from build123d import *
from build123d.topology import SkipClean

# Parameters (mm, degrees)
SKETCH1_R                 = 13.75
SKETCH1_R_2               = 6
BOSS_EXTRUDE1_DEPTH       = 12
SKETCH2_R                 = 13.75
SKETCH2_R_2               = 4.01
BOSS_EXTRUDE3_DEPTH       = 10.98
SKETCH3_R                 = 30
BOSS_EXTRUDE4_DEPTH       = 11.02
F_4_0MM_DOWEL_HOLE1_D     = 4
F_4_0MM_DOWEL_HOLE1_DEPTH = 25.4
F_4_0MM_DOWEL_HOLE1_TIP   = 1.201721238
SKETCH11_W                = 4.05
SKETCH11_H                = 4.3
CUT_EXTRUDE1_DEPTH        = 10
CUT_EXTRUDE2_START        = -32
SKETCH15_R                = 4.01
CUT_EXTRUDE2_DEPTH        = 32
SKETCH16_R                = 13.810706785
SKETCH16_R_2              = 3.943549935
BOSS_EXTRUDE5_DEPTH       = 11


with BuildPart() as part:
    # Sketch1 → Boss-Extrude1 (new body)
    with BuildSketch(Plane(origin=(0, 0, 0), x_dir=(0, 0, -1), z_dir=(1, 0, 0))):
        Circle(SKETCH1_R)
        Circle(SKETCH1_R_2, mode=Mode.SUBTRACT)
    extrude(amount=BOSS_EXTRUDE1_DEPTH)

    # Sketch2 → Boss-Extrude3 (add)
    with BuildSketch(Plane(origin=(12, 0, 0), x_dir=(0, 0, -1), z_dir=(1, 0, 0))):
        with Locations(Location((0, 0, 0), (0, 0, 180))):
            Circle(SKETCH2_R)
        with Locations(Location((0, 0, 0), (0, 0, 180))):
            Circle(SKETCH2_R_2, mode=Mode.SUBTRACT)
    extrude(amount=BOSS_EXTRUDE3_DEPTH)

    # Sketch3 → Boss-Extrude4 (add)
    with BuildSketch(Plane(origin=(22.98, 0, 0), x_dir=(0, 0, -1), z_dir=(1, 0, 0))):
        with Locations(Location((0, 0, 0), (0, 0, 180))):
            Circle(SKETCH3_R)
    extrude(amount=BOSS_EXTRUDE4_DEPTH)

    # Ø4.0mm Dowel Hole1
    with Locations(Plane(origin=(34, 0, 0), x_dir=(0, 0, -1), z_dir=(1, 0, 0))):
        with Locations((-21.643670313, 10.843162234), (-2.353154811, 24.568381237), (19.178491269, 14.724914261), (21.419621846, -8.843771717), (-19.402539736, -12.725523744), (2.129106344, -22.56899072)):
            Hole(F_4_0MM_DOWEL_HOLE1_D / 2, depth=F_4_0MM_DOWEL_HOLE1_DEPTH)
            with Locations((0, 0, -(F_4_0MM_DOWEL_HOLE1_DEPTH + F_4_0MM_DOWEL_HOLE1_TIP / 2))):  # 118° drill point
                Cone(0, F_4_0MM_DOWEL_HOLE1_D / 2, F_4_0MM_DOWEL_HOLE1_TIP, mode=Mode.SUBTRACT)

    # Sketch11 → Cut-Extrude1 (cut)
    with BuildSketch(Plane.ZY):
        with Locations((0, 6)):
            Rectangle(SKETCH11_W, SKETCH11_H)
    extrude(amount=-CUT_EXTRUDE1_DEPTH, mode=Mode.SUBTRACT)

    # Sketch14 → Ø4.0mm Dowel Hole2 (revolve, cut)
    with BuildSketch(Plane(origin=(5, 8.15, 0), x_dir=(0, 0, -1), z_dir=(1, 0, 0))):
        Polygon((0, 0), (0, 26.601721238), (2, 25.4), (2, 0), align=None)
    revolve(axis=Axis((5, 1.8, 0), (0, 1, 0)), mode=Mode.SUBTRACT)

    # Sketch15 → Cut-Extrude2 (cut)
    with SkipClean():  # the faces are left unmerged after this step: merging them gives an invalid solid
        with BuildSketch(Plane(origin=(34, 0, 0), x_dir=(0, 0, -1), z_dir=(1, 0, 0)).offset(CUT_EXTRUDE2_START)):
            Circle(SKETCH15_R)
        extrude(amount=CUT_EXTRUDE2_DEPTH, mode=Mode.SUBTRACT)
    add(part.part.scale(1), mode=Mode.REPLACE)  # the faces are merged on a copy

    # Sketch16 → Boss-Extrude5 (add)
    with BuildSketch(Plane(origin=(34, 0, 0), x_dir=(0, 0, -1), z_dir=(1, 0, 0))):
        with Locations(Location((0, 0, 0), (0, 0, 180))):
            Circle(SKETCH16_R)
        with Locations(Location((0, 0.056450065, 0), (0, 0, 180))):
            Circle(SKETCH16_R_2, mode=Mode.SUBTRACT)
    extrude(amount=BOSS_EXTRUDE5_DEPTH)


solid = part.part
Geometry check sheet. Reference: the model listing, model coordinates, mm. A direction names the side the tool comes from. Round coordinates to 2 decimals unless told otherwise and drop trailing zeros. Loops run counter-clockwise (first coordinate to the right, second up) from the corner with the lowest first, then second, coordinate; pieces in that order, holes last. Notation, with made-up numbers: (20, 13.5) -> (45, 13.5) arc R20 ccw to (45, 30.5) -> close; hole circle Ø3 at (58, 45). An arc over 180 degrees is marked (long way). Answer as a JSON object with one key per item and string values. Group by question number.
Item 1: Cross-section at D-D, the plane y = 18. Record the cut outline in (x, z), plus the area to 3 significant figures.
Item 2: Thickness scan on line 1 along Y through (x, z) = (28.5, -20); line 2 along X through (y, z) = (10.75, 0); line 3 along Y through (x, z) = (25, -2). Record the ranges inside material, lowest first.
Item 3: Release check for a two-part mould opening along Y. For faces 5 (the face through (28.4, -7.5, -22.9)), 6 (the face through (3.8, 8.15, -1.8)), 7 (the face through (22.98, 0, -14)), 8 (the face through (39.423, -4.148, 13.173)) record: pulls with the +Y half, pulls with the -Y half, needs draft (parallel to the pull), parting line crosses it, or undercut.
Item 4: Cross-section at B-B, the plane x = 5. Record the cut outline in (y, z) (3 decimals), plus the area to 3 significant figures.
Item 5: Cross-section at A-A, the plane z = -22. Record the cut outline in (x, y).
Item 6: Cross-section at C-C, the plane x = 19. Record the cut outline in (y, z).
Item 7: Set-up check for faces 1 (the face through (7, 11, 0)), 2 (the face through (45, 3, 3)), 3 (the face through (34, 13, 6)), 4 (the face through (10, 7, 0)): record each of +Z, -Z, +X, -X, +Y, -Y from which the full face is reachable in a straight line by a thin tool's end or side.
Item 8: Depth check by flat-ended pin: pin 1 Ø4 at (y, z) = (3.5, 20.5) entering from +X; pin 2 Ø3 at (x, z) = (3.5, 1) entering from -Y; pin 3 Ø1.3 at (x, y) = (3, 6.5) entering from +Z. Enter the tip coordinate at first touch or a pass-through.
Determined:
{
 "1": {"outline": "(22.98, -24) -> (34, -24) -> (34, 24) -> (22.98, 24) -> close", "area": "529 mm²"},
 "2": {"line 1": "y = -22.36 to -10.25, -7.43 to 12.9, 16.55 to 22.36", "line 2": "x = 0 to 3, 7 to 45", "line 3": "y = -29.93 to -24.56, -20.57 to -3.48, 3.48 to 29.93"},
 "3": {"face 5": "undercut", "face 6": "undercut", "face 7": "needs draft", "face 8": "parting line crosses it"},
 "4": {"outline": "(5.648, -2.025) arc R6 cw (long way) to (5.648, 2.025) -> (8.15, 2.025) -> (8.15, 2) -> (13.604, 2) arc R13.75 ccw (long way) to (13.604, -2) -> (8.15, -2) -> (8.15, -2.025) -> close", "area": "449 mm²"},
 "5": {"outline": "(22.98, -20.4) -> (34, -20.4) -> (34, -10.76) -> (22.98, -10.76) -> close; (22.98, -6.93) -> (34, -6.93) -> (34, 20.4) -> (22.98, 20.4) -> close"},
 "6": {"outline": "circle Ø27.5 at (0, 0); hole circle Ø8.02 at (0, 0)"},
 "7": {"face 1": "+Y", "face 2": "+Z, -Z, +X, +Y, -Y", "face 3": "+X", "face 4": "-X"},
 "8": {"pin 1": "stops at x = 34", "pin 2": "stops at y = -13.75", "pin 3": "stops at z = 12.44"}
}
